Autodesk Inventor part; units mm, degrees
ref_plane "YZ Plane" through (0, 0, 0) normal (1, 0, 0) x (0, 1, 0)
ref_plane "XZ Plane" through (0, 0, 0) normal (0, 1, 0) x (-1, 0, 0)
ref_plane "XY Plane" through (0, 0, 0) normal (0, 0, 1) x (1, 0, 0)
sketch "Sketch1" plane through (0, 0, 0) normal (0, 1, 0) x (-1, 0, 0)
  line L0 (0, -2.7135) -> (-2.35, -1.3568)
  line L1 (-2.35, -1.3568) -> (-2.35, 1.3568)
  line L2 (-2.35, 1.3568) -> (0, 2.7135)
  line L3 (0, 2.7135) -> (2.35, 1.3568)
  line L4 (2.35, 1.3568) -> (2.35, -1.3568)
  line L5 (2.35, -1.3568) -> (0, -2.7135)
  circle A0 centre (0, 0) radius 1.5
  dimension "d1" = 3
  dimension "d4" = 4.7
extrude "Extrusion1" add sketch "Sketch1" along normal blind 60
sketch "Sketch2" plane through (0, 0, 0) normal (0, -1, 0) x (1, 0, 0)
  circle A0 centre (0, 0) radius 1.5
  circle A1 centre (0, 0) radius 1.5
  dimension "d5" = 3
extrude "Extrusion2" add sketch "Sketch2" along normal blind 6 and the other way blind 4
thread "Thread1"
properties part number "Brass Spacer" material "Brass, Soft Yellow"
The model under review builds one solid part; all positions refer to its coordinate system, in mm. A direction names the side the tool comes from. Give positions to 0.01 mm unless a question says otherwise; leave off trailing zeros. Order: outer loops, then holes, each group sorted by start corner. A loop starts at its lowest first (then second) coordinate and runs counter-clockwise, first axis right, second up. Notation, with made-up numbers: M -12,77 L 14,77 A22 ccw 14,86 Z; hole C 31.25,30 d1. An arc over 180 degrees is marked long. One line per question, with ' | ' between items. Start each with the question number.
1) Mouldability with a two-part tool opening along Z and no side actions: class faces 3 (the face through (0, 4, 0)), 4 (the face through (1.5, 31.61, -0.07)), 5 (the face through (2.35, 30, 0)), 6 (the face through (-1.159, 29.58, 2.045)) as pulls with the +Z half, pulls with the -Z half, needs draft (parallel to the pull), parting line crosses it, or undercut.
2) Wall thickness on L1, parallel to X at y = 20, z = 0; L2, parallel to Z at x = 0, y = 19; L3, parallel to Y at x = 0.4, z = 0.3: over which ranges is each line inside the solid? List them lowest first. Write a range as from..to.
3) For faces 1 (the face through (-1.5, -2.96, -0.07)), 2 (the face through (1.191, 29.58, 2.026)), list the 3-axis set-ups (+Z, -Z, +X, -X, +Y, -Y) from which the entire face can be reached by the end or side of a thin tool; tool diameter is ignored.
4) Consider section A-A, the plane y = 46. Give the boundary of the cut face in (x, z).
5) Consider section B-B, the plane z = 0. Give the boundary of the cut face in (x, y), then the cut area to 3 significant figures.
6) Clearance check with flat-ended pins moving along their axes: P1, Ø2, axis at y = 47.5, z = 2, coming from the +X side; P2, Ø1, axis at x = 1, z = 2, coming from the -Y side; P3, Ø0.9, axis at x = -0.5, z = 0, coming from the +Y side. State where each tip first meets the part, or that it passes through.
7) Consider section C-C, the plane x = 0.65. Give the boundary of the cut face in (y, z), then the cut area to 3 significant figures.
Found:
1) face 3: undercut | face 4: undercut | face 5: needs draft | face 6: pulls with the +Z half
2) L1: x = -2.35..-1.5, 1.5..2.35 | L2: z = -2.71..-1.5, 1.5..2.71 | L3: y = -6..4
3) face 1: -Y | face 2: +Z, +X, +Y, -Y
4) outline: M -2.35,-1.36 L 0,-2.71 L 2.35,-1.36 L 2.35,1.36 L 0,2.71 L -2.35,1.36 Z; hole C 0,0 d3
5) outline: M -2.35,0 L -1.5,0 L -1.5,-6 L 1.5,-6 L 1.5,0 L 2.35,0 L 2.35,60 L 1.5,60 L 1.5,4 L -1.5,4 L -1.5,60 L -2.35,60 Z | area: 132 mm²
6) P1: stops at x = 2.35 | P2: stops at y = 0 | P3: stops at y = 4
7) outline: M -6,-1.35 L 0,-1.35 L 0,-2.34 L 60,-2.34 L 60,-1.35 L 4,-1.35 L 4,1.35 L 60,1.35 L 60,2.34 L 0,2.34 L 0,1.35 L -6,1.35 Z | area: 145 mm²
